Geometry check sheet. Reference: the model listing, model coordinates, mm. Give positions to 0.01 mm unless a question says otherwise; leave off trailing zeros. Write each loop counter-clockwise with the first axis right and the second up, starting at its lowest first coordinate (ties: lowest second). Pieces come first, ordered by that corner, then holes. Notation, with made-up numbers: (20, -7.75) -> (41, -7.75) arc R20 ccw to (41, 12.25) -> close; hole circle Ø10 at (-31, 66.25). An arc over 180 degrees is marked (long way). One line per item, written item: value.
from build123d import *

# Parameters (mm, degrees)
SKETCH1_R           = 2
SKETCH1_W           = 15
SKETCH1_H           = 5
SKETCH1_W_2         = 61.5
SKETCH1_H_2         = 61.5
SKETCH1_R_2         = 4
SKETCH1_R_3         = 6
SKETCH1_W_3         = 30
SKETCH1_H_3         = 20
SKETCH1_W_4         = 12
SKETCH1_H_4         = 4.5
BOSS_EXTRUDE1_DEPTH = 5


with BuildPart() as part:
    # Sketch1 → Boss-Extrude1 (new body)
    with BuildSketch(Plane.XY):
        Polygon((148, -50), (168, -50), (168, -30), (163, -30), (163, 30), (168, 30), (168, 50), (148, 50), (148, 55), (98, 55), (98, 50), (50, 50), (50, 55), (-50, 55), (-50, 50), (-98, 50), (-98, 55), (-148, 55), (-148, 50), (-168, 50), (-168, 30), (-163, 30), (-163, -30), (-168, -30), (-168, -50), (-148, -50), (-148, -55), (-98, -55), (-98, -50), (-50, -50), (-50, -55), (50, -55), (50, -50), (98, -50), (98, -55), (148, -55), align=None)
        with Locations((-20, -35.75)):
            Circle(SKETCH1_R, mode=Mode.SUBTRACT)
        with Locations((-65, -22.5)):
            Rectangle(SKETCH1_W, SKETCH1_H, mode=Mode.SUBTRACT)
        with Locations((51.5, -35.75)):
            Circle(SKETCH1_R, mode=Mode.SUBTRACT)
        with Locations((71.5, -35.75)):
            Circle(SKETCH1_R, mode=Mode.SUBTRACT)
        with Locations((143, -35.75)):
            Circle(SKETCH1_R, mode=Mode.SUBTRACT)
        with Locations((15.75, 0)):
            Rectangle(SKETCH1_W_2, SKETCH1_H_2, mode=Mode.SUBTRACT)
        with Locations((-135, 0)):
            Circle(SKETCH1_R_2, mode=Mode.SUBTRACT)
        with Locations((-110, 0)):
            Circle(SKETCH1_R_3, mode=Mode.SUBTRACT)
        with Locations((-65, 0)):
            Rectangle(SKETCH1_W_3, SKETCH1_H_3, mode=Mode.SUBTRACT)
        with Locations((-65, 22.25)):
            Rectangle(SKETCH1_W_4, SKETCH1_H_4, mode=Mode.SUBTRACT)
        with Locations((-20, 35.75)):
            Circle(SKETCH1_R, mode=Mode.SUBTRACT)
        with Locations((107.25, 0)):
            Rectangle(SKETCH1_W_2, SKETCH1_H_2, mode=Mode.SUBTRACT)
        with Locations((51.5, 35.75)):
            Circle(SKETCH1_R, mode=Mode.SUBTRACT)
        with Locations((71.5, 35.75)):
            Circle(SKETCH1_R, mode=Mode.SUBTRACT)
        with Locations((143, 35.75)):
            Circle(SKETCH1_R, mode=Mode.SUBTRACT)
    extrude(amount=BOSS_EXTRUDE1_DEPTH)


solid = part.part
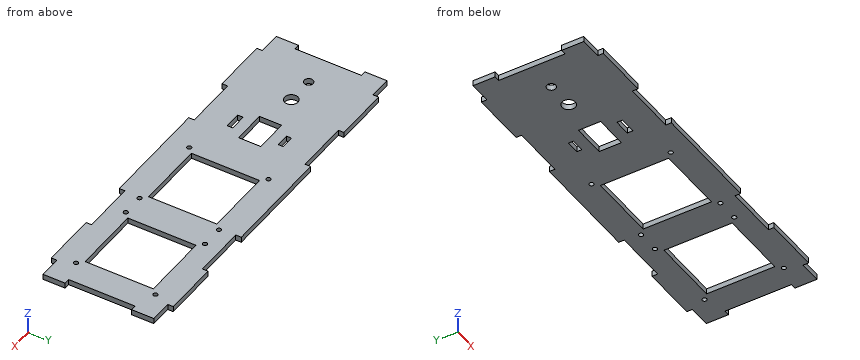
1) Sectioned sample at C-C on y = -15. Record the cut outline in (x, z), plus the area to 4 significant figures.
Verdict:
outline: (-163, 0) -> (-15, 0) -> (-15, 5) -> (-163, 5) -> close; (46.5, 0) -> (76.5, 0) -> (76.5, 5) -> (46.5, 5) -> close; (138, 0) -> (163, 0) -> (163, 5) -> (138, 5) -> close
area: 1,015 mm^2
2) Scan lines: probe 1 along Y at (x, z) = (-20, 2.4); probe 2 along X at (y, z) = (-36, 1.25); probe 3 along Y at (x, z) = (71.5, 1). Record each from-to range of solid material in increasing order.
Verdict:
probe 1: -55 to -37.75, -33.75 to 33.75, 37.75 to 55
probe 2: -168 to -21.98, -18.02 to 49.52, 53.48 to 69.52, 73.48 to 141.02, 144.98 to 168
probe 3: -50 to -37.75, -33.75 to 33.75, 37.75 to 50
3) Sectioned sample at A-A on x = 121. Record the cut outline in (y, z), plus the area to 4 significant figures.
Verdict:
outline: (-55, 0) -> (-30.75, 0) -> (-30.75, 5) -> (-55, 5) -> close; (30.75, 0) -> (55, 0) -> (55, 5) -> (30.75, 5) -> close
area: 242.5 mm^2
4) Sectioned sample at B-B on y = 0. Record the cut outline in (x, z), plus the area to 3 significant figures.
Verdict:
outline: (-163, 0) -> (-139, 0) -> (-139, 5) -> (-163, 5) -> close; (-131, 0) -> (-116, 0) -> (-116, 5) -> (-131, 5) -> close; (-104, 0) -> (-80, 0) -> (-80, 5) -> (-104, 5) -> close; (-50, 0) -> (-15, 0) -> (-15, 5) -> (-50, 5) -> close; (46.5, 0) -> (76.5, 0) -> (76.5, 5) -> (46.5, 5) -> close; (138, 0) -> (163, 0) -> (163, 5) -> (138, 5) -> close
area: 765 mm^2
5) Depth check by flat-ended pin: pin 1 Ø1.5 at (x, z) = (-64.5, 4) entering from -Y; pin 2 Ø2.5 at (x, z) = (-71, 1.5) entering from +Y; pin 3 Ø2.5 at (y, z) = (52.5, 3.5) entering from -X. Enter the tip coordinate at first touch or a pass-through.
Verdict:
pin 1: y = -50
pin 2: y = 50
pin 3: x = -148
6) Sectioned sample at D-D on x = -110. Record the cut outline in (y, z).
Verdict:
outline: (-55, 0) -> (-6, 0) -> (-6, 5) -> (-55, 5) -> close; (6, 0) -> (55, 0) -> (55, 5) -> (6, 5) -> close
